```python
from build123d import *

# Parameters (mm, degrees)
F0_W     = 101.6
F0_H     = 101.6
F1_DEPTH = 177.8
F2_R     = 31.75
F3_DEPTH = 88.9
F4_R     = 6.35
F5_R     = 5.08


with BuildPart() as f1:
    # F0 (on Front) → F1 (new body)
    with BuildSketch(Plane.XZ):
        with Locations((-43.596539, 12.358267)):
            Rectangle(F0_W, F0_H)
    extrude(amount=-F1_DEPTH)

    # F2 (on face) → F3 (join)
    with BuildSketch(Plane.XZ):
        with Locations((-43.596539, 12.358267)):
            Circle(F2_R)
    extrude(amount=F3_DEPTH)

    # F4
    f4_edges = [f1.edges().sort_by_distance(p)[0] for p in [
        (7.203461, 0, 12.358267),
        (-94.396539, 0, 12.358267),
        (7.203461, 177.8, 12.358267),
        (-94.396539, 177.8, 12.358267),
    ]]
    fillet(f4_edges, radius=F4_R)

    # F5
    f5_edges = [f1.edges().sort_by_distance(p)[0] for p in [
        (7.203461, 88.9, 63.158267),
    ]]
    fillet(f5_edges, radius=F5_R)


solid = f1.part
```
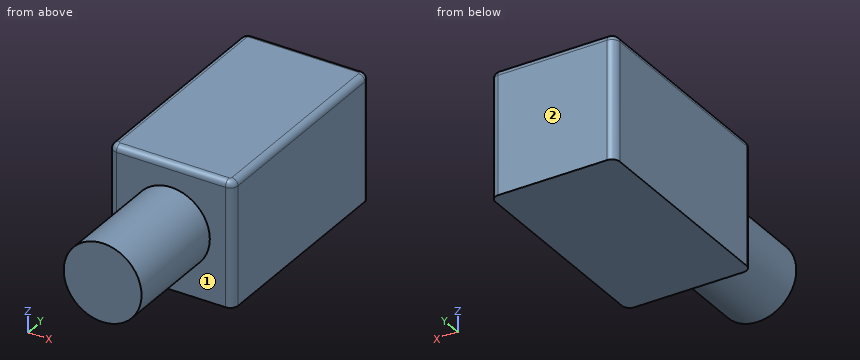
Source: CAD feature listing. Evaluate the final solid. Frame: model axes, mm. Face numbers are marked on the shaded views. A direction names the side the tool comes from. Give positions to 0.01 mm unless a question says otherwise; leave off trailing zeros. Loops run counter-clockwise (first coordinate to the right, second up) from the corner with the lowest first, then second, coordinate; pieces in that order, holes last. Notation, with made-up numbers: (-30.75, 46.5) -> (15.25, 46.5) arc R12 cw to (15.25, 53.5) -> close; hole circle Ø1 at (19, 22). An arc over 180 degrees is marked (long way). Use a Markdown table: item, result. Add a question column.
(1) Ray query, line 1 (Y direction, x = -85, z = 28); line 2 (Z direction, x = -44.5, y = -44); line 3 (X direction, y = -36, z = -5). Return the intervals inside material, ascending.
(2) Section query B-B (x = -42). Output: boundary loops of the cut face in (y, z).
(3) First-contact query: pin 1 Ø12 at (y, z) = (-32, -22.5) entering from +X. Flat tip, straight axial feed; report the tip coordinate or a pass-through.
(4) Section query C-C (y = -72). Output: boundary loops of the cut face in (x, z).
(5) Access query for the marked faces 1 and 2. Directions: +Z, -Z, +X, -X, +Y, -Y. A direction counts if a zero-diameter tool reaches every point of the face in a straight line with its end or side. Return the directions, or none.
(6) Section query D-D (z = -9.5). Output: boundary loops of the cut face in (x, y).
(7) Section query A-A (z = -25.5). Output: boundary loops of the cut face in (x, y).
Checked values:
| question | item | result |
|---|---|---|
| 1 | line 1 | 0 to 177.8 |
| 1 | line 2 | -19.38 to 44.1 |
| 1 | line 3 | -70.18 to -17.01 |
| 2 | outline | (-88.9, -19.35) -> (0, -19.35) -> (0, -38.44) -> (177.8, -38.44) -> (177.8, 58.08) arc R5.08 ccw to (172.72, 63.16) -> (5.08, 63.16) arc R5.08 ccw to (0, 58.08) -> (0, 44.07) -> (-88.9, 44.07) -> close |
| 3 | pin 1 | x = -30.36 |
| 4 | outline | circle Ø63.5 at (-43.6, 12.36) |
| 5 | face 1 | -Y |
| 5 | face 2 | +Z, -Z, +X, -X, +Y |
| 6 | outline | (-94.4, 6.35) arc R6.35 ccw to (-88.05, 0) -> (-66.62, 0) -> (-66.62, -88.9) -> (-20.57, -88.9) -> (-20.57, 0) -> (0.85, 0) arc R6.35 ccw to (7.2, 6.35) -> (7.2, 171.45) arc R6.35 ccw to (0.85, 177.8) -> (-88.05, 177.8) arc R6.35 ccw to (-94.4, 171.45) -> close |
| 7 | outline | (-94.4, 6.35) arc R6.35 ccw to (-88.05, 0) -> (0.85, 0) arc R6.35 ccw to (7.2, 6.35) -> (7.2, 171.45) arc R6.35 ccw to (0.85, 177.8) -> (-88.05, 177.8) arc R6.35 ccw to (-94.4, 171.45) -> close |
